Autodesk Inventor part; units mm, degrees
ref_plane "YZ Plane" through (0, 0, 0) normal (1, 0, 0) x (0, 1, 0)
ref_plane "XZ Plane" through (0, 0, 0) normal (0, 1, 0) x (-1, 0, 0)
ref_plane "XY Plane" through (0, 0, 0) normal (0, 0, 1) x (1, 0, 0)
sketch "Эскиз1" plane through (0, 0, 0) normal (1, 0, 0) x (0, 1, 0)
  circle A0 centre (0, 0) radius 5
  line L0 (0, -2.5) -> (2.5037, 0)
  line L1 (2.5037, 0) -> (0, 2.5074)
  line L2 (0, 2.5074) -> (-2.5037, 0.0074)
  line L3 (-2.5037, 0.0074) -> (0, -2.5)
extrude "Выдавливание1" add sketch "Эскиз1" along normal blind 6
chamfer "Фаска1" distance 6 distance2 2 1 edges at (6, -5, 0) measured on face at (4, 4.9353, -0.8021)
ref_plane "РабПлоскость3" through (0, 0, 5.25) normal (0, 0, 1) x (1, 0, 0)
sketch "Эскиз5" plane through (0, 0, 5.25) normal (0, 0, 1) x (1, 0, 0)
  line L0 (0, 1) -> (2.4, 0)
  line L1 (2.4, 0) -> (2.4, -2)
  line L2 (2.4, -2) -> (1.6636, -2.3125)
  line L3 (0, 1) -> (1.6636, -2.3125)
  point P0 (0, 0)
extrude "Выдавливание2" add sketch "Эскиз5" along normal blind 19 draft -2 and the other way blind 2
pattern_circular "Круговой массив1" count 4 over 360 about axis through (3, 0, 0) along (1, 0, 0) of "Выдавливание2"
sketch "Эскиз6" plane through (0, 0, 0) normal (0, 1, 0) x (-1, 0, 0)
  line L0 (-1.1407, -15.27) -> (6.3977, -15.27)
  line L1 (6.3977, -15.27) -> (6.3977, 15.5226)
  line L2 (6.3977, 15.5226) -> (-1.1407, 15.5226)
  line L3 (-1.1407, 15.5226) -> (-1.1407, -15.27)
  point P0 (0, 0)
extrude "Выдавливание3" cut sketch "Эскиз6" along normal through all both and the other way through all
sketch "Эскиз7" plane through (0, 0, 0) normal (0, 1, 0) x (-1, 0, 0)
  line L0 (-1.4062, -24.2443) -> (6.1599, -24.2443)
  line L1 (6.1599, -24.2443) -> (6.1599, 24.4007)
  line L2 (6.1599, 24.4007) -> (-1.4062, 24.4007)
  line L3 (-1.4062, 24.4007) -> (-1.4062, -24.2443)
  point P0 (0, 0)
extrude "Выдавливание4" cut sketch "Эскиз7" along normal through all both and the other way through all
properties part number "Нож"
Could you check a few things on this model? Use its own coordinates, in mm. A direction names the side the tool comes from. Round coordinates to 2 decimals unless told otherwise and drop trailing zeros. Loops run counter-clockwise (first coordinate to the right, second up) from the corner with the lowest first, then second, coordinate; pieces in that order, holes last. Notation, with made-up numbers: (84.25, 25) - (102.25, 25) arc R35 ccw to (102.25, 58) - close; hole circle Ø5 at (45.5, 24.5). An arc over 180 degrees is marked (long way). Write item = value, one per line.
1) If we mould it in two halves opening along Y, with no side actions, what happens to faces 6 (the flat face through (2.4, -5, -1)), 7 (the flat face through (3.7, -1.3, -1.2))? For each: pulls with the +Y half, pulls with the -Y half, needs draft (parallel to the pull), parting line crosses it, or undercut.
Computed:
face_6 = needs draft
face_7 = undercut
2) Imagine slicing it at C-C (y = -17). Please give me the cut outline in (x, z).
Computed:
outline = (1.41, -0.89) - (1.86, -1.78) - (1.99, -1.73) - (1.99, -0.27) - (1.41, -0.03) - close
3) I need wall thicknesses on line 1 along X through (y, z) = (1.5, -2.5); line 2 along Z through (x, y) = (3.8, -2); line 3 along Y through (x, z) = (1.6, -0.5). Which ranges of each line are inside material? Lowest first, please. Write a range as from..to.
Computed:
line_1 = 1.41..6
line_2 = -3.15..-0.5, 0.51..3.15
line_3 = -24.25..-2, 2..4.44
4) Imagine slicing it at A-A (x = 4.45). Please give me the cut outline in (y, z).
Computed:
outline = circle Ø7.03 at (0, 0); hole (-2.5, 0.01) - (0, -2.5) - (2.5, 0) - (0, 2.51) - close
5) I'm going to push flat-ended pins straight in: P1, Ø1, axis at x = 4.5, y = -7, coming from the -Z side; P2, Ø1.5, axis at x = 3.5, y = 2.5, coming from the +Z side; P3, Ø1, axis at y = -2, z = 12, coming from the -X side; P4, Ø1.5, axis at x = 3, z = -5, coming from the -Y side. Where does each tip first touch, or does it pass through?
Computed:
P1 = through
P2 = 3.5
P3 = 1.52
P4 = -0.06
6) On a 3-axis mill with a long thin cutter (end or side, diameter ignored), from which of +Z, -Z, +X, -X, +Y, -Y can I reach the whole of each face in a straight line? I mean faces 1 (the flat face through (1.406, 2, 2)), 2 (the flat face through (3.7, 1.2, -1.3)), 3 (the flat face through (2.4, 5, 1)), 4 (the flat face through (2.4, 1, -5)), 5 (the flat face through (2.4, -1, 5)). Say none if no direction works.
Computed:
face_1 = +Z, -Z, -X, +Y, -Y
face_2 = +X, -X
face_3 = +Z, +X, +Y
face_4 = -Z, +X, +Y
face_5 = +Z, +X, -Y
